CAD build for the part. Positions are in the model's coordinates, mm. A direction names the side the tool comes from. Round coordinates to 2 decimals unless told otherwise and drop trailing zeros. Loops run counter-clockwise (first coordinate to the right, second up) from the corner with the lowest first, then second, coordinate; pieces in that order, holes last. Notation, with made-up numbers: M -23.75,7.5 L 0.25,7.5 A20 ccw 0.25,32.5 Z; hole C -15.75,-39 d1. An arc over 180 degrees is marked long. Put each result on its own line as item: value. Start each with the question number.
from build123d import *

# Parameters (mm, degrees)
F0_W     = 63.5
F0_H     = 12.319
F1_DEPTH = 19.05
F2_W     = 51.562
F2_H     = 2.9845
F3_DEPTH = 25.4
F4_W     = 7.7978
F4_H     = 1.778
F5_DEPTH = 9.525
F6_R     = 1.5875
F7_DEPTH = 25.4
F8_R     = 1.27


with BuildPart() as f1:
    # F0 (on Top) → F1 (new body)
    with BuildSketch(Plane.XY):
        Rectangle(F0_W, F0_H)
    extrude(amount=F1_DEPTH)

    # F2 (on face) → F3 (cut)
    with BuildSketch(Plane.XY.offset(19.05)):
        Polygon((24.981306, -6.1595), (25.781, -3.175), (-25.781, -3.175), (-24.981306, -6.1595), (0, -6.1595), align=None)
        with Locations((0, -1.68275)):
            Rectangle(F2_W, F2_H)
    extrude(amount=-F3_DEPTH, mode=Mode.SUBTRACT)

    # F4 (on face) → F5 (cut)
    with BuildSketch(Plane.XY.offset(19.05)):
        with Locations((0, -0.1905)):
            Rectangle(F4_W, F4_H)
    extrude(amount=-F5_DEPTH, mode=Mode.SUBTRACT)

    # F6 (on face) → F7 (cut)
    with BuildSketch(Plane.XZ.offset(0.1905)):
        with Locations((0, 15.113)):
            Circle(F6_R)
    extrude(amount=-F7_DEPTH, mode=Mode.SUBTRACT)

    # F8
    f8_edges = [f1.edges().sort_by_distance(p)[0] for p in [
        (31.75, 6.1595, 9.525),
        (-31.75, 0, 0),
        (-31.75, -6.1595, 9.525),
        (31.75, -6.1595, 9.525),
        (31.75, 0, 0),
        (-31.75, 0, 19.05),
        (31.75, 0, 19.05),
        (-31.75, 6.1595, 9.525),
    ]]
    fillet(f8_edges, radius=F8_R)


solid = f1.part
(1) Drill centre lines: line 1 along X through (y, z) = (-2.5, 13.25); line 2 along Z through (x, y) = (0, 3.2); line 3 along Y through (x, z) = (9, 3.75). Where is each one in solid material? Low to high.
(2) Cut at C-C on y = -4.25. List the corners of the cut face in (x, z).
(3) Mould opens along Z. For faces 1 (the cylindrical face through (-31.388, 0.086, 0.382)), 2 (the cylindrical face through (-31.388, -5.778, 9.658)), 3 (the cylindrical face through (0.853, 3.391, 16.452)) say: +Z half, -Z half, draft (parallel to the pull), parting line (faces both ways), or undercut.
(4) Tool access for faces 4 (the flat face through (0, 0.698, 13)), 5 (the flat face through (28, -6.16, 9)), 6 (the flat face through (-25.781, -2, 10)): list every direction of +Z, -Z, +X, -X, +Y, -Y with a clear straight run to the whole face (end or side of a thin tool).
(5) Flat gauge pins, fed straight in: pin 1 Ø2.5 at (x, z) = (-0.5, 14) entering from -Y; pin 2 Ø0.7 at (x, y) = (-1, 0) entering from +Z (3 decimals); pin 3 Ø1 at (x, z) = (14.5, 11.5) entering from -Y. Where does each tip first touch, or does it go through?
Taken from the geometry:
1. line 1: -31.75 to -25.78, 25.78 to 31.75
1. line 2: 0 to 13.53, 16.7 to 19.05
1. line 3: -0.19 to 6.16
2. outline: M -31.75,1.27 A1.27 ccw -30.48,0 L -25.49,0 L -25.49,19.05 L -30.48,19.05 A1.27 ccw -31.75,17.78 Z; M 25.49,0 L 30.48,0 A1.27 ccw 31.75,1.27 L 31.75,17.78 A1.27 ccw 30.48,19.05 L 25.49,19.05 Z
3. face 1: -Z half
3. face 2: draft
3. face 3: undercut
4. face 4: +Z, -Y
4. face 5: +Z, -Z, +X, -X, -Y
4. face 6: +Z, -Z
5. pin 1: y = 0.7
5. pin 2: z = 9.525
5. pin 3: y = -0.19
